Here's how the part is built. I have some questions about the finished solid (model axes, mm). A direction names the side the tool comes from. Round coordinates to 2 decimals unless told otherwise and drop trailing zeros. Write each loop counter-clockwise with the first axis right and the second up, starting at its lowest first coordinate (ties: lowest second). Pieces come first, ordered by that corner, then holes. Notation, with made-up numbers: (-30, 24.5) -> (23, 24.5) arc R20 ccw to (23, 49.5) -> close; hole circle Ø8 at (-35.5, 12.25). An arc over 180 degrees is marked (long way). Answer in a Markdown table with one row per item.
from build123d import *

# Parameters (mm, degrees)
BOSS_EXTRUDE2_DEPTH = 5
FILLET8_R           = 65
SKETCH4_R           = 2
SKETCH4_R_2         = 1.5621
SKETCH4_R_3         = 1.55575
SKETCH4_R_4         = 1.6
CUT_EXTRUDE1_DEPTH  = 5
FILLET9_R           = 5
FILLET10_R          = 5


with BuildPart() as part:
    # Sketch1 → Boss-Extrude2 (new body)
    with BuildSketch(Plane(origin=(0, 0, 0), x_dir=(1, 0, 0), z_dir=(0, 1, 0))):
        Polygon((65.5, 80), (-65.5, 80), (-65.5, -7), (-60.15, -7), (-60.15, -83.5), (60.15, -83.5), (60.15, -7), (65.5, -7), align=None)
    extrude(amount=BOSS_EXTRUDE2_DEPTH)

    # Fillet8
    fillet8_edges = [part.edges().sort_by_distance(p)[0] for p in [
        (-65.5, 2.5, -80),
        (65.5, 2.5, -80),
    ]]
    fillet(fillet8_edges, radius=FILLET8_R)

    # Sketch4 → Cut-Extrude1 (cut)
    with BuildSketch(Plane(origin=(0, 5, 0), x_dir=(1, 0, 0), z_dir=(0, 1, 0))):
        with Locations(Location((43.047144734, 55.54428083, 0), (0, 0, 270))):
            Circle(SKETCH4_R)
        with Locations(Location((-43.047144734, 55.54428083, 0), (0, 0, 90))):
            Circle(SKETCH4_R)
        with Locations(Location((-53.249046458, -73.796312774, 0), (0, 0, 270))):
            Circle(SKETCH4_R)
        with Locations(Location((53.249046458, -73.796312774, 0), (0, 0, 90))):
            Circle(SKETCH4_R)
        with Locations(Location((-35.41902795, 50.193626152, 0), (0, 0, 270))):
            Circle(SKETCH4_R_2)
        with Locations(Location((39.71417205, 50.193626152, 0), (0, 0, 270))):
            Circle(SKETCH4_R_2)
        with Locations(Location((-35.41902795, 1.857426152, 0), (0, 0, 270))):
            Circle(SKETCH4_R_2)
        with Locations(Location((47.20717205, 1.857426152, 0), (0, 0, 270))):
            Circle(SKETCH4_R_2)
        with Locations(Location((-7.869013511, -50.333617588, 0), (0, 0, 270))):
            Circle(SKETCH4_R_3)
        with Locations(Location((7.688486489, -50.333617588, 0), (0, 0, 270))):
            Circle(SKETCH4_R_3)
        with Locations(Location((40.071563944, 40.662108402, 0), (0, 0, 270))):
            Circle(SKETCH4_R_4)
        with Locations(Location((40.071563944, 9.662108402, 0), (0, 0, 270))):
            Circle(SKETCH4_R_4)
        with Locations(Location((-20.928436056, 40.662108402, 0), (0, 0, 270))):
            Circle(SKETCH4_R_4)
        with Locations(Location((-20.928436056, 9.662108402, 0), (0, 0, 270))):
            Circle(SKETCH4_R_4)
        with Locations(Location((52.65, -33.659925039, 0), (0, 0, 270))):
            Circle(SKETCH4_R_4)
        with Locations(Location((52.65, -44.659925039, 0), (0, 0, 270))):
            Circle(SKETCH4_R_4)
        with Locations(Location((52.65, -55.659925039, 0), (0, 0, 270))):
            Circle(SKETCH4_R_4)
        with Locations(Location((-52.65, -55.659925039, 0), (0, 0, 90))):
            Circle(SKETCH4_R_4)
        with Locations(Location((-52.65, -44.659925039, 0), (0, 0, 90))):
            Circle(SKETCH4_R_4)
        with Locations(Location((-52.65, -33.659925039, 0), (0, 0, 90))):
            Circle(SKETCH4_R_4)
        with BuildLine():
            Line((-25.229195822, 57.914440008), (31.548032439, 57.914440008))
            ThreePointArc((31.548032439, 57.914440008), (33.918191616, 55.54428083), (31.548032439, 53.174121653))
            Line((31.548032439, 53.174121653), (-25.229195822, 53.174121653))
            ThreePointArc((-25.229195822, 53.174121653), (-27.599355, 55.54428083), (-25.229195822, 57.914440008))
        make_face()
        with BuildLine():
            Line((-15.471860298, -0.8868659), (43.047144734, -0.8868659))
            ThreePointArc((43.047144734, -0.8868659), (45.750426625, -3.590147791), (43.047144734, -6.293429682))
            Line((43.047144734, -6.293429682), (-15.471860298, -6.293429682))
            ThreePointArc((-15.471860298, -6.293429682), (-18.175142189, -3.590147791), (-15.471860298, -0.8868659))
        make_face()
        with BuildLine():
            Line((57.484245228, 35.149431205), (57.484245228, 6.868248507))
            ThreePointArc((57.484245228, 6.868248507), (55.106623673, 4.490626953), (52.729002119, 6.868248507))
            Line((52.729002119, 6.868248507), (52.729002119, 35.149431205))
            ThreePointArc((52.729002119, 35.149431205), (55.106623673, 37.52705276), (57.484245228, 35.149431205))
        make_face()
        with BuildLine():
            Line((-51.995557855, -9.38715687), (-43.754184302, -9.38715687))
            ThreePointArc((-43.754184302, -9.38715687), (-40.74405673, -12.397284441), (-43.754184302, -15.407412013))
            Line((-43.754184302, -15.407412013), (-51.995557855, -15.407412013))
            ThreePointArc((-51.995557855, -15.407412013), (-55.005685427, -12.397284441), (-51.995557855, -9.38715687))
        make_face()
        with BuildLine():
            Line((51.995557855, -9.38715687), (43.754184302, -9.38715687))
            ThreePointArc((43.754184302, -9.38715687), (40.74405673, -12.397284441), (43.754184302, -15.407412013))
            Line((43.754184302, -15.407412013), (51.995557855, -15.407412013))
            ThreePointArc((51.995557855, -15.407412013), (55.005685427, -12.397284441), (51.995557855, -9.38715687))
        make_face()
        with BuildLine():
            Line((-48.684552143, 12.171246466), (-48.684552143, 2.805296047))
            ThreePointArc((-48.684552143, 2.805296047), (-53.249046458, -1.759198268), (-57.813540773, 2.805296047))
            Line((-57.813540773, 2.805296047), (-57.813540773, 12.171246466))
            ThreePointArc((-57.813540773, 12.171246466), (-53.249046458, 16.73574078), (-48.684552143, 12.171246466))
        make_face()
    extrude(amount=-CUT_EXTRUDE1_DEPTH, mode=Mode.SUBTRACT)

    # Fillet9
    fillet9_edges = [part.edges().sort_by_distance(p)[0] for p in [
        (60.15, 2.5, 83.5),
        (-60.15, 2.5, 83.5),
        (-65.5, 2.5, 7),
        (65.5, 2.5, 7),
    ]]
    fillet(fillet9_edges, radius=FILLET9_R)

    # Fillet10
    fillet10_edges = [part.edges().sort_by_distance(p)[0] for p in [
        (60.15, 2.5, 7),
        (-60.15, 2.5, 7),
    ]]
    fillet(fillet10_edges, radius=FILLET10_R)


solid = part.part
1) I want a section at B-B, the plane z = 18. List the corners of the cut face in (x, y) for me.
Response:
| item | result |
|---|---|
| outline | (-60.15, 0) -> (60.15, 0) -> (60.15, 5) -> (-60.15, 5) -> close |
2) I want a section at D-D, the plane z = -64.5. List the corners of the cut face in (x, y) for me.
Response:
| item | result |
|---|---|
| outline | (-42.63, 0) -> (42.63, 0) -> (42.63, 5) -> (-42.63, 5) -> close |
3) Which directions (+Z, -Z, +X, -X, +Y, -Y) give clear straight access to the entire face, cutting with the end or side of a thin tool? Please do faces 4 (the face through (-48, 3, 15.407)), 5 (the face through (-1, 5, 19)).
Response:
| item | result |
|---|---|
| face 4 | +Y, -Y |
| face 5 | +Z, -Z, +X, -X, +Y |
4) For pin 1 (5 mm diameter, centred on x = -43.05, z = -55.54, fed in from +Y); pin 2 (1 mm diameter, centred on x = 6, y = 3.5, fed in from -Z); pin 3 (2.5 mm diameter, centred on x = 3.5, y = 1.5, fed in from -Z); pin 4 (3 mm diameter, centred on y = 3.5, z = 54.5, fed in from -X), each with a flat end and sliding along its axis, tell me the tip position at first contact or that it passes through.
Response:
| item | result |
|---|---|
| pin 1 | stops at y = 5 |
| pin 2 | stops at z = -79.81 |
| pin 3 | stops at z = -79.98 |
| pin 4 | stops at x = -60.15 |
5) I want a section at C-C, the plane y = 1.1. Count the separate pieces of the cut face and the enclosed holes in it, and give its area (3 significant figures).
Response:
| item | result |
|---|---|
| separate pieces | 1 |
| enclosed holes | 26 |
| area | 17,500 mm^2 |
6) I want a section at A-A, the plane z = -20.5. List the corners of the cut face in (x, y) for me, and give its area (3 significant figures).
Response:
| item | result |
|---|---|
| outline | (-65.27, 0) -> (52.73, 0) -> (52.73, 5) -> (-65.27, 5) -> close; (57.48, 0) -> (65.27, 0) -> (65.27, 5) -> (57.48, 5) -> close |
| area | 629 mm^2 |
7) I need wall thicknesses on line 1 (X direction, y = 0.35, z = 56); line 2 (Z direction, x = 43.5, y = 4.65); line 3 (Z direction, x = 46, y = 0.8). Which ranges of each line are inside material? Lowest first, please. Write a range as [from, to].
Response:
| item | result |
|---|---|
| line 1 | x = [-60.15, -54.21], [-51.09, 51.09], [54.21, 60.15] |
| line 2 | z = [-63.74, -57.49], [-53.6, 0.93], [6.26, 9.4], [15.4, 83.5] |
| line 3 | z = [-61.42, -2.85], [-0.87, 9.39], [15.41, 83.5] |
8) We'd pull the mould along Z, two halves only. Please class faces 1 (the face through (4, 3, -53.174)), 2 (the face through (-1, 2, 83.5)), 3 (the face through (-1, 0, 19)): +Z half, -Z half, draft (parallel to the pull), parting line (faces both ways), or undercut.
Response:
| item | result |
|---|---|
| face 1 | undercut |
| face 2 | +Z half |
| face 3 | draft |
